from build123d import *

# Parameters (mm, degrees)
F0_R     = 3.175
F1_DEPTH = 1.5875


with BuildPart() as f1:
    # F0 (on Front) → F1 (new body, symmetric)
    with BuildSketch(Plane.XZ):
        with BuildLine():
            Line((18.2378478348, 0), (3.175, 0))
            ThreePointArc((3.175, 0), (0, -3.175), (-3.175, 0))
            Line((-3.175, 0), (-18.2378478348, 0))
            ThreePointArc((-18.2378478348, 0), (-12.9826090881, -1.5809399099), (-9.4718777788, -5.7989573302))
            Line((-9.4718777788, -5.7989573302), (0, -10.7457929799))
            Line((0, -10.7457929799), (3.3629814094, -8.9894235763))
            ThreePointArc((3.3629814094, -8.9894235763), (4.4455137358, -7.0979565161), (6.4924834296, -6.35))
            Line((6.4924834296, -6.35), (8.4167772684, -6.35))
            Line((8.4167772684, -6.35), (9.4718777788, -5.7989573302))
            ThreePointArc((9.4718777788, -5.7989573302), (12.9826090881, -1.5809399099), (18.2378478348, 0))
        make_face()
        with BuildLine():
            ThreePointArc((20.1887122983, -0.2019236384), (19.2184911582, -0.0506153935), (18.2378478348, 0))
            ThreePointArc((18.2378478348, 0), (12.9826090881, -1.5809399099), (9.4718777788, -5.7989573302))
            Line((9.4718777788, -5.7989573302), (20.1887122983, -0.2019236384))
        make_face()
        with BuildLine():
            ThreePointArc((-9.4718777788, -5.7989573302), (-12.9826090881, -1.5809399099), (-18.2378478348, 0))
            ThreePointArc((-18.2378478348, 0), (-19.2184911582, -0.0506153935), (-20.1887122983, -0.2019236384))
            Line((-20.1887122983, -0.2019236384), (-9.4718777788, -5.7989573302))
        make_face()
        with BuildLine():
            ThreePointArc((22.6472823333, -1.082102843), (21.4483041232, -0.5573584248), (20.1887122983, -0.2019236384))
            Line((20.1887122983, -0.2019236384), (9.4718777788, -5.7989573302))
            ThreePointArc((9.4718777788, -5.7989573302), (9.3604581347, -6.0728156028), (9.2575917138, -6.35))
            Line((9.2575917138, -6.35), (18.2378478348, -6.35))
            ThreePointArc((18.2378478348, -6.35), (20.4829118651, -7.2799359697), (21.4128478348, -9.525))
            ThreePointArc((21.4128478348, -9.525), (20.4829118651, -11.7700640303), (18.2378478348, -12.7))
            Line((18.2378478348, -12.7), (9.2575917138, -12.7))
            ThreePointArc((9.2575917138, -12.7), (11.0435001343, -15.7673542165), (13.8284133364, -17.967897157))
            ThreePointArc((13.8284133364, -17.967897157), (15.9677124226, -18.7755194562), (18.2378478348, -19.05))
            ThreePointArc((18.2378478348, -19.05), (24.9730399256, -16.2601920908), (27.7628478348, -9.525))
            ThreePointArc((27.7628478348, -9.525), (26.384181016, -4.5891231072), (22.6472823333, -1.082102843))
        make_face()
        with BuildLine():
            ThreePointArc((9.2575917138, -6.35), (9.3604581347, -6.0728156028), (9.4718777788, -5.7989573302))
            Line((9.4718777788, -5.7989573302), (8.4167772684, -6.35))
            Line((8.4167772684, -6.35), (9.2575917138, -6.35))
        make_face()
        with BuildLine():
            Line((0, -10.7457929799), (-9.4718777788, -5.7989573302))
            ThreePointArc((-9.4718777788, -5.7989573302), (-8.9045341204, -7.6237161947), (-8.7128478348, -9.525))
            ThreePointArc((-8.7128478348, -9.525), (-10.0915146536, -14.4608768928), (-13.8284133364, -17.967897157))
            Line((-13.8284133364, -17.967897157), (0, -10.7457929799))
        make_face()
        with BuildLine():
            ThreePointArc((-8.7128478348, -9.525), (-8.9045341204, -7.6237161947), (-9.4718777788, -5.7989573302))
            Line((-9.4718777788, -5.7989573302), (-20.1887122983, -0.2019236384))
            ThreePointArc((-20.1887122983, -0.2019236384), (-20.7031117187, -0.3245598484), (-21.2099123798, -0.4755548601))
            ThreePointArc((-21.2099123798, -0.4755548601), (-21.9410366156, -0.7493508585), (-22.6472823333, -1.082102843))
            ThreePointArc((-22.6472823333, -1.082102843), (-27.7308527221, -10.3050533377), (-21.2099123798, -18.5744451399))
            ThreePointArc((-21.2099123798, -18.5744451399), (-19.7427830564, -18.9303599069), (-18.2378478348, -19.05))
            ThreePointArc((-18.2378478348, -19.05), (-15.9677124226, -18.7755194562), (-13.8284133364, -17.967897157))
            ThreePointArc((-13.8284133364, -17.967897157), (-10.0915146536, -14.4608768928), (-8.7128478348, -9.525))
        make_face()
        with Locations((-18.2378478348, -9.525)):
            Circle(F0_R, mode=Mode.SUBTRACT)
        with BuildLine():
            Line((13.8284133364, -17.967897157), (0, -10.7457929799))
            Line((0, -10.7457929799), (-13.8284133364, -17.967897157))
            ThreePointArc((-13.8284133364, -17.967897157), (-15.9677124226, -18.7755194562), (-18.2378478348, -19.05))
            Line((-18.2378478348, -19.05), (18.2378478348, -19.05))
            ThreePointArc((18.2378478348, -19.05), (15.9677124226, -18.7755194562), (13.8284133364, -17.967897157))
        make_face()
        with BuildLine():
            Line((3.3629814094, -8.9894235763), (0, -10.7457929799))
            Line((0, -10.7457929799), (13.8284133364, -17.967897157))
            ThreePointArc((13.8284133364, -17.967897157), (11.0435001343, -15.7673542165), (9.2575917138, -12.7))
            Line((9.2575917138, -12.7), (6.4924834296, -12.7))
            ThreePointArc((6.4924834296, -12.7), (4.0654399457, -11.5719696938), (3.3629814094, -8.9894235763))
        make_face()
        with BuildLine():
            Line((-22.6472823333, -1.082102843), (-21.9535177998, -0.7197735133))
            Line((-21.9535177998, -0.7197735133), (-39.097144814, -6.3501702098))
            Line((-39.097144814, -6.3501702098), (-39.097144814, -12.6998297902))
            Line((-39.097144814, -12.6998297902), (-21.2099123798, -18.5744451399))
            ThreePointArc((-21.2099123798, -18.5744451399), (-27.7308527221, -10.3050533377), (-22.6472823333, -1.082102843))
        make_face()
    extrude(amount=F1_DEPTH, both=True)


solid = f1.part
Input: part model. Units: mm. Frame: model coordinates. Give positions to 0.01 mm unless a question says otherwise; leave off trailing zeros. Order: outer loops, then holes, each group sorted by start corner. A loop starts at its lowest first (then second) coordinate and runs counter-clockwise, first axis right, second up. Notation, with made-up numbers: (14.25, -33.5) - (60.25, -33.5) arc R23 ccw to (60.25, -2.5) - close; hole circle Ø3 at (3.5, 73.5). An arc over 180 degrees is marked (long way). Write each question's results on one line, items separated by ' | '.
Item 1: Material intervals for line 1 along X through (y, z) = (-0.85, -9.25); line 2 along X through (y, z) = (-0.8, -6.75); line 3 along Z through (x, y) = (12.5, 0.35), sorted ascending.
A:
line 1: x = -39.1 to -21.4, -15.07 to 3.33, 21.4 to 27.76 | line 2: x = -39.1 to -19.78, -16.7 to 4.95, 19.78 to 27.35 | line 3: z = -19.05 to -12.7, -6.35 to 0
Item 2: Section C-C (y = -1). Return loops of the section in (x, z) (3 decimals), and give its area (3 significant figures).
A:
outline: (-39.097, -12.7) - (-21.21, -18.574) arc R9.525 ccw to (-18.238, -19.05) - (18.238, -19.05) arc R9.525 ccw to (18.238, 0) - (3.175, 0) arc R3.175 cw to (-3.175, 0) - (-18.238, 0) arc R9.525 ccw to (-22.647, -1.082) - (-21.954, -0.72) - (-39.097, -6.35) - close; hole circle Ø6.35 at (-18.238, -9.525); hole (6.492, -12.7) - (18.238, -12.7) arc R3.175 ccw to (18.238, -6.35) - (6.492, -6.35) arc R3.175 ccw to start | area: 958 mm^2
Item 3: Section D-D (x = 10.5). Return loops of the section in (y, z).
A:
outline: (-1.59, -19.05) - (1.59, -19.05) - (1.59, -12.7) - (-1.59, -12.7) - close; (-1.59, -6.35) - (1.59, -6.35) - (1.59, 0) - (-1.59, 0) - close
Item 4: Contact query for flat-ended pins moving along their axis: pin 1 Ø8.5 at (x, z) = (-18.24, -9.52) entering from +Y; pin 2 Ø1 at (y, z) = (1, -8.5) entering from +X. Output: stop coordinate, or through.
A:
pin 1: stops at y = 1.59 | pin 2: stops at x = 27.75
Item 5: Draft query along X for faces 1 (the flat face through (-6, -1.588, -9)), 2 (the cylindrical face through (0.07, -0.022, -3.174)). Return one class per face: released by +X, released by -X, zero draft, split by the parting line, or undercut.
A:
face 1: zero draft | face 2: undercut
Item 6: Section B-B (z = -8.25). Return loops of the section in (x, y).
A:
outline: (-39.1, -1.59) - (-21.15, -1.59) - (-21.15, 1.59) - (-39.1, 1.59) - close; (-15.33, -1.59) - (3.58, -1.59) - (3.58, 1.59) - (-15.33, 1.59) - close; (21.15, -1.59) - (27.68, -1.59) - (27.68, 1.59) - (21.15, 1.59) - close
Item 7: Section A-A (x = -17). Return loops of the section in (y, z).
A:
outline: (-1.59, -19.05) - (1.59, -19.05) - (1.59, -12.45) - (-1.59, -12.45) - close; (-1.59, -6.6) - (1.59, -6.6) - (1.59, 0) - (-1.59, 0) - close
